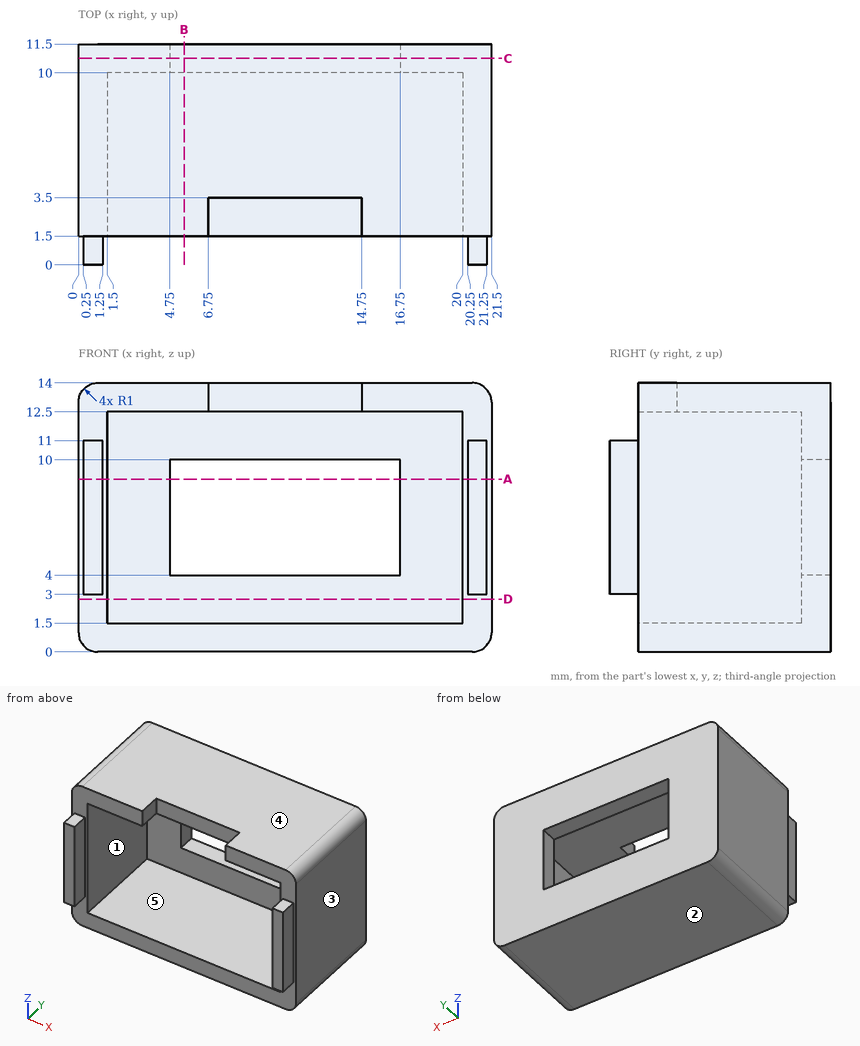
Here's the drawing with two shaded views (mm, measured from the low corner). I have some questions. A direction names the side the tool comes from. Give positions to 0.01 mm unless a question says otherwise; leave off trailing zeros. Loops run counter-clockwise (first coordinate to the right, second up) from the corner with the lowest first, then second, coordinate; pieces in that order, holes last. Notation, with made-up numbers: (45, -7.5) - (86, -7.5) arc R18 ccw to (86, 7.5) - close; hole circle Ø5 at (79, -38). An arc over 180 degrees is marked (long way). Return JSON: item names as keys, results as strings.
1. I want a section at D-D on z = 2.75. Please give me the cut outline in (x, y).
Output values:
{"outline": "(0, 1.5) - (1.5, 1.5) - (1.5, 10) - (20, 10) - (20, 1.5) - (21.5, 1.5) - (21.5, 11.5) - (0, 11.5) - close"}
2. For the marked faces 4 and 5, which set-ups out of +Z, -Z, +X, -X, +Y, -Y let a thin tool reach every point of the face, with its end or its side?
Output values:
{"face 4": "+Z, +X, -X, +Y, -Y", "face 5": "-Y"}
3. If I drill on line 1 (Z direction, x = 9.5, y = 7.75); line 2 (X direction, y = 7.75, z = 9); line 3 (Y direction, x = 9, z = 2.75), over which ranges is the centre line in solid material (lowest first)?
Output values:
{"line 1": "z = 0 to 1.5, 12.5 to 14", "line 2": "x = 0 to 1.5, 20 to 21.5", "line 3": "y = 10 to 11.5"}
4. I want a section at A-A on z = 9. Please give me the cut outline in (x, y).
Output values:
{"outline": "(0, 1.5) - (0.25, 1.5) - (0.25, 0) - (1.25, 0) - (1.25, 1.5) - (1.5, 1.5) - (1.5, 10) - (4.75, 10) - (4.75, 11.5) - (0, 11.5) - close; (16.75, 10) - (20, 10) - (20, 1.5) - (20.25, 1.5) - (20.25, 0) - (21.25, 0) - (21.25, 1.5) - (21.5, 1.5) - (21.5, 11.5) - (16.75, 11.5) - close"}
5. I want a section at B-B on x = 5.5. Please give me the cut outline in (y, z).
Output values:
{"outline": "(1.5, 0) - (11.5, 0) - (11.5, 4) - (10, 4) - (10, 1.5) - (1.5, 1.5) - close; (1.5, 12.5) - (10, 12.5) - (10, 10) - (11.5, 10) - (11.5, 14) - (1.5, 14) - close"}
6. We'd pull the mould along Z, two halves only. Please class the marked faces 1, 2 and 3: +Z half, -Z half, draft (parallel to the pull), parting line (faces both ways), or undercut.
Output values:
{"face 1": "undercut", "face 2": "-Z half", "face 3": "draft"}
7. I want a section at C-C on y = 10.75. Please give me the cut outline in (x, z).
Output values:
{"outline": "(0, 1) arc R1 ccw to (1, 0) - (20.5, 0) arc R1 ccw to (21.5, 1) - (21.5, 13) arc R1 ccw to (20.5, 14) - (1, 14) arc R1 ccw to (0, 13) - close; hole (4.75, 4) - (16.75, 4) - (16.75, 10) - (4.75, 10) - close"}
8. I'm going to push flat-ended pins straight in: pin 1 Ø1.1 at (x, y) = (20.5, 0.5) entering from +Z; pin 2 Ø6 at (x, y) = (9.5, 3) entering from -Z; pin 3 Ø1.6 at (x, z) = (9, 13) entering from -Y; pin 4 Ø1.2 at (y, z) = (0.5, 6) entering from +X. Where does each tip first touch, or does it pass through?
Output values:
{"pin 1": "stops at z = 11", "pin 2": "stops at z = 0", "pin 3": "stops at y = 3.5", "pin 4": "stops at x = 21.25"}
